Autodesk Inventor part; units mm, degrees
ref_plane "YZ Plane" through (0, 0, 0) normal (1, 0, 0) x (0, 1, 0)
ref_plane "XZ Plane" through (0, 0, 0) normal (0, 1, 0) x (-1, 0, 0)
ref_plane "XY Plane" through (0, 0, 0) normal (0, 0, 1) x (1, 0, 0)
sketch "Эскиз1" plane through (0, 0, 0) normal (0, 0, 1) x (1, 0, 0)
  line L0 (0, 0) -> (74.2, 0)
  line L1 (0, 0) -> (0, 9.2)
  line L2 (0, 9.2) -> (6, 9.2)
  line L3 (6, 9.2) -> (6, 6.2)
  line L4 (6, 6.2) -> (3, 6.2)
  line L5 (3, 6.2) -> (3, 3)
  line L6 (71.2, 3) -> (71.2, 6.2)
  line L7 (71.2, 6.2) -> (68.2, 6.2)
  line L8 (68.2, 6.2) -> (68.2, 9.2)
  line L9 (68.2, 9.2) -> (74.2, 9.2)
  line L10 (74.2, 9.2) -> (74.2, 0)
  line L11 (3, 3) -> (71.2, 3)
  dimension "d2" = 68.2
  dimension "d3" = 3
  dimension "d4" = 3
  dimension "d5" = 3
  dimension "d6" = 3
  dimension "d7" = 3
  dimension "d8" = 3
  dimension "d9" = 3
  dimension "d10" = 3.2
extrude "Выдавливание1" add sketch "Эскиз1" along normal blind 35
sketch "Эскиз2" plane through (0, 0, 0) normal (0, -1, 0) x (1, 0, 0)
  line L0 (6, 0) -> (0, 0)
  line L1 (0, 0) -> (74.2, 0)
  line L2 (74.2, 0) -> (74.2, -3)
  line L3 (74.2, -3) -> (0, -3)
  line L4 (0, -3) -> (0, 0)
  point P0 (74.2, -1.5)
  dimension "d13" = 3
extrude "Выдавливание2" add sketch "Эскиз2" against normal blind 25
sketch "Эскиз3" plane through (0, 25, 0) normal (0, 0, 1) x (1, 0, 0)
  line L0 (74.2, -15.8) -> (74.2, 0)
  line L1 (74.2, -15.8) -> (74.2, 0)
  line L2 (0, 0) -> (74.2, 0)
  line L3 (74.2, 0) -> (0, 0)
  line L4 (6, -15.8) -> (0, -15.8)
  line L5 (0, 0) -> (0, -15.8)
  line L6 (0, -15.8) -> (6, -15.8)
  line L7 (6, -15.8) -> (6, -3)
  line L8 (6, -3) -> (68.2, -3)
  line L9 (68.2, -3) -> (68.2, -15.8)
  line L10 (74.2, -15.8) -> (68.2, -15.8)
  line L11 (74.2, -15.8) -> (68.2, -15.8)
  point P0 (0, -25)
  dimension "d16" = 3
extrude "Выдавливание3" add sketch "Эскиз3" along normal blind 2
properties part number "креплениедлякамерыверх"
Source: CAD feature listing. Evaluate the final solid. Frame: model axes, mm. A direction names the side the tool comes from. Give positions to 0.01 mm unless a question says otherwise; leave off trailing zeros. Order: outer loops, then holes, each group sorted by start corner. A loop starts at its lowest first (then second) coordinate and runs counter-clockwise, first axis right, second up.
(1) Section query C-C (z = 14). Return the cut outline in (x, y).
(2) Contact query for flat-ended pins moving along their axis: P1, Ø3, axis at y = 11, z = 22.5, coming from the -X side; P2, Ø5, axis at x = 3, z = 11.5, coming from the +Y side; P3, Ø15, axis at x = 36, y = 13, coming from the +Z side; P4, Ø6, axis at x = 22.5, z = 16, coming from the +Y side. Output: stop coordinate, or through.
(3) Section query D-D (y = 4). Return the cut outline in (x, z), plus the area to 3 significant figures.
(4) Section query A-A (x = 69). Return the cut outline in (y, z), plus the area to 3 significant figures.
(5) Section query B-B (y = 15.5). Return the cut outline in (x, z), plus the area to 3 significant figures.
(6) Pull-direction query (X, two-part tool) for faces 1 (the face through (37, 0, 16)), 2 (the face through (37, 3, 17)), 3 (the face through (0, 7, 12)); classes: +X half, -X half, draft (parallel to the pull), parting line (faces both ways), or undercut.
(7) Material intervals for line 1 along X through (y, z) = (8, 17); line 2 along Y through (x, z) = (12, 0.5); line 3 along Z through (x, y) = (46, 13.25), sorted ascending.
(8) Access query for faces 4 (the face through (71, 9.2, 18)), 5 (the face through (5, 6.2, 17)), 6 (the face through (74.2, 7, 12)). Directions: +Z, -Z, +X, -X, +Y, -Y. A direction counts if a zero-diameter tool reaches every point of the face in a straight line with its end or side. Return the directions, or none.
Outcome:
1. outline: (0, 0) - (74.2, 0) - (74.2, 9.2) - (68.2, 9.2) - (68.2, 6.2) - (71.2, 6.2) - (71.2, 3) - (3, 3) - (3, 6.2) - (6, 6.2) - (6, 9.2) - (0, 9.2) - close
2. P1: passes through
2. P2: stops at y = 9.2
2. P3: stops at z = 0
2. P4: stops at y = 3
3. outline: (0, -3) - (74.2, -3) - (74.2, 35) - (71.2, 35) - (71.2, 0) - (3, 0) - (3, 35) - (0, 35) - close
3. area: 433 mm2
4. outline: (0, -3) - (25, -3) - (25, 2) - (9.2, 2) - (9.2, 35) - (6.2, 35) - (6.2, 0) - (3, 0) - (3, 35) - (0, 35) - close
4. area: 317 mm2
5. outline: (0, -3) - (74.2, -3) - (74.2, 2) - (68.2, 2) - (68.2, 0) - (6, 0) - (6, 2) - (0, 2) - close
5. area: 247 mm2
6. face 1: draft
6. face 2: undercut
6. face 3: -X half
7. line 1: x = 0 to 6, 68.2 to 74.2
7. line 2: y = 0 to 3, 22 to 25
7. line 3: z = -3 to 0
8. face 4: +Z, +X, -X, +Y
8. face 5: +Z
8. face 6: +Z, -Z, +X, +Y, -Y
